Work out the finished part from the listing and answer in its coordinate system (mm). Give positions to 0.01 mm unless a question says otherwise; leave off trailing zeros. Order: outer loops, then holes, each group sorted by start corner. A loop starts at its lowest first (then second) coordinate and runs counter-clockwise, first axis right, second up. Notation, with made-up numbers: (10, 11.5) -> (49, 11.5) arc R9 ccw to (49, 15.5) -> close; hole circle Ø1 at (18.5, -20). An arc over 180 degrees is marked (long way). Answer as CSV lines item,"result". Start each with the question number.
1. For a pull along Y with two mould halves and no side action, classify faces 1 (the flat face through (110, -9, 1.016)), 2 (the flat face through (12, 29, 0.508)) as released by +Y, released by -Y, zero draft, split by the parting line, or undercut.
2. Find the intervals of material crossed by L1, parallel to Y at x = 28.5, z = 0.55; L2, parallel to Z at x = 58, y = 4, in increasing order.
3. A flat-ended cylindrical pin translates along its axis: pin 1 (0.6 mm diameter, centred on x = -53.5, z = 1, fed in from -Y). Find the tip coordinate at first contact, or state that the pin passes through.
4. A cutting plane is placed at B-B (z = 0.7). State how many separate pieces and enclosed holes the cut face has, then the cut area to 3 significant figures.
5. A cutting plane is placed at A-A (x = -7.5). Give the vertices of the cut face in (y, z), then the cut area to 3 significant figures.
from build123d import *

# Parameters (mm, degrees)
F0_W     = 226.06
F0_H     = 142.24
F0_W_2   = 25.4
F0_H_2   = 25.4
F1_DEPTH = 0.508
F2_DEPTH = 1.016


with BuildPart() as f1:
    # F0 (on Top) → F1 (new body)
    with BuildSketch(Plane.XY):
        with Locations((12.174503, 18.332164)):
            Rectangle(F0_W, F0_H)
        with Locations((-85.615497, -37.547836)):
            Rectangle(F0_W_2, F0_H_2, mode=Mode.SUBTRACT)
        with Locations((-57.675497, -37.547836)):
            Rectangle(F0_W_2, F0_H_2, mode=Mode.SUBTRACT)
        with Locations((-29.735497, -37.547836)):
            Rectangle(F0_W_2, F0_H_2, mode=Mode.SUBTRACT)
        with Locations((-1.795497, -37.547836)):
            Rectangle(F0_W_2, F0_H_2, mode=Mode.SUBTRACT)
        with Locations((-85.615497, -9.607836)):
            Rectangle(F0_W_2, F0_H_2, mode=Mode.SUBTRACT)
        with Locations((-57.675497, -9.607836)):
            Rectangle(F0_W_2, F0_H_2, mode=Mode.SUBTRACT)
        with Locations((-85.615497, 18.332164)):
            Rectangle(F0_W_2, F0_H_2, mode=Mode.SUBTRACT)
        with Locations((-57.675497, 18.332164)):
            Rectangle(F0_W_2, F0_H_2, mode=Mode.SUBTRACT)
        with Locations((-29.735497, -9.607836)):
            Rectangle(F0_W_2, F0_H_2, mode=Mode.SUBTRACT)
        with Locations((-1.795497, -9.607836)):
            Rectangle(F0_W_2, F0_H_2, mode=Mode.SUBTRACT)
        with Locations((-29.735497, 18.332164)):
            Rectangle(F0_W_2, F0_H_2, mode=Mode.SUBTRACT)
        with Locations((-1.795497, 18.332164)):
            Rectangle(F0_W_2, F0_H_2, mode=Mode.SUBTRACT)
        with Locations((26.144503, -37.547836)):
            Rectangle(F0_W_2, F0_H_2, mode=Mode.SUBTRACT)
        with Locations((54.084503, -37.547836)):
            Rectangle(F0_W_2, F0_H_2, mode=Mode.SUBTRACT)
        with Locations((82.024503, -37.547836)):
            Rectangle(F0_W_2, F0_H_2, mode=Mode.SUBTRACT)
        with Locations((109.964503, -37.547836)):
            Rectangle(F0_W_2, F0_H_2, mode=Mode.SUBTRACT)
        with Locations((26.144503, -9.607836)):
            Rectangle(F0_W_2, F0_H_2, mode=Mode.SUBTRACT)
        with Locations((54.084503, -9.607836)):
            Rectangle(F0_W_2, F0_H_2, mode=Mode.SUBTRACT)
        with Locations((26.144503, 18.332164)):
            Rectangle(F0_W_2, F0_H_2, mode=Mode.SUBTRACT)
        with Locations((54.084503, 18.332164)):
            Rectangle(F0_W_2, F0_H_2, mode=Mode.SUBTRACT)
        with Locations((82.024503, -9.607836)):
            Rectangle(F0_W_2, F0_H_2, mode=Mode.SUBTRACT)
        with Locations((109.964503, -9.607836)):
            Rectangle(F0_W_2, F0_H_2, mode=Mode.SUBTRACT)
        with Locations((82.024503, 18.332164)):
            Rectangle(F0_W_2, F0_H_2, mode=Mode.SUBTRACT)
        with Locations((109.964503, 18.332164)):
            Rectangle(F0_W_2, F0_H_2, mode=Mode.SUBTRACT)
        with Locations((-85.615497, 46.272164)):
            Rectangle(F0_W_2, F0_H_2, mode=Mode.SUBTRACT)
        with Locations((-57.675497, 46.272164)):
            Rectangle(F0_W_2, F0_H_2, mode=Mode.SUBTRACT)
        with Locations((-29.735497, 46.272164)):
            Rectangle(F0_W_2, F0_H_2, mode=Mode.SUBTRACT)
        with Locations((-1.795497, 46.272164)):
            Rectangle(F0_W_2, F0_H_2, mode=Mode.SUBTRACT)
        with Locations((-85.615497, 74.212164)):
            Rectangle(F0_W_2, F0_H_2, mode=Mode.SUBTRACT)
        with Locations((-57.675497, 74.212164)):
            Rectangle(F0_W_2, F0_H_2, mode=Mode.SUBTRACT)
        with Locations((-29.735497, 74.212164)):
            Rectangle(F0_W_2, F0_H_2, mode=Mode.SUBTRACT)
        with Locations((-1.795497, 74.212164)):
            Rectangle(F0_W_2, F0_H_2, mode=Mode.SUBTRACT)
        with Locations((26.144503, 46.272164)):
            Rectangle(F0_W_2, F0_H_2, mode=Mode.SUBTRACT)
        with Locations((54.084503, 46.272164)):
            Rectangle(F0_W_2, F0_H_2, mode=Mode.SUBTRACT)
        with Locations((82.024503, 46.272164)):
            Rectangle(F0_W_2, F0_H_2, mode=Mode.SUBTRACT)
        with Locations((109.964503, 46.272164)):
            Rectangle(F0_W_2, F0_H_2, mode=Mode.SUBTRACT)
        with Locations((26.144503, 74.212164)):
            Rectangle(F0_W_2, F0_H_2, mode=Mode.SUBTRACT)
        with Locations((54.084503, 74.212164)):
            Rectangle(F0_W_2, F0_H_2, mode=Mode.SUBTRACT)
        with Locations((82.024503, 74.212164)):
            Rectangle(F0_W_2, F0_H_2, mode=Mode.SUBTRACT)
        with Locations((109.964503, 74.212164)):
            Rectangle(F0_W_2, F0_H_2, mode=Mode.SUBTRACT)
    extrude(amount=F1_DEPTH)

    # F0 (on Top) → F2 (join)
    with BuildSketch(Plane.XY):
        with Locations((-85.615497, 18.332164)):
            Rectangle(F0_W_2, F0_H_2)
        with Locations((-57.675497, 18.332164)):
            Rectangle(F0_W_2, F0_H_2)
        with Locations((-57.675497, 46.272164)):
            Rectangle(F0_W_2, F0_H_2)
        with Locations((-85.615497, 46.272164)):
            Rectangle(F0_W_2, F0_H_2)
        with Locations((-85.615497, 74.212164)):
            Rectangle(F0_W_2, F0_H_2)
        with Locations((-57.675497, 74.212164)):
            Rectangle(F0_W_2, F0_H_2)
        with Locations((-85.615497, -9.607836)):
            Rectangle(F0_W_2, F0_H_2)
        with Locations((-57.675497, -9.607836)):
            Rectangle(F0_W_2, F0_H_2)
        with Locations((-57.675497, -37.547836)):
            Rectangle(F0_W_2, F0_H_2)
        with Locations((-85.615497, -37.547836)):
            Rectangle(F0_W_2, F0_H_2)
        with Locations((-29.735497, -37.547836)):
            Rectangle(F0_W_2, F0_H_2)
        with Locations((-29.735497, -9.607836)):
            Rectangle(F0_W_2, F0_H_2)
        with Locations((-29.735497, 18.332164)):
            Rectangle(F0_W_2, F0_H_2)
        with Locations((-29.735497, 46.272164)):
            Rectangle(F0_W_2, F0_H_2)
        with Locations((-29.735497, 74.212164)):
            Rectangle(F0_W_2, F0_H_2)
        with Locations((-1.795497, 74.212164)):
            Rectangle(F0_W_2, F0_H_2)
        with Locations((-1.795497, 46.272164)):
            Rectangle(F0_W_2, F0_H_2)
        with Locations((-1.795497, 18.332164)):
            Rectangle(F0_W_2, F0_H_2)
        with Locations((-1.795497, -9.607836)):
            Rectangle(F0_W_2, F0_H_2)
        with Locations((-1.795497, -37.547836)):
            Rectangle(F0_W_2, F0_H_2)
        with Locations((26.144503, -37.547836)):
            Rectangle(F0_W_2, F0_H_2)
        with Locations((26.144503, -9.607836)):
            Rectangle(F0_W_2, F0_H_2)
        with Locations((26.144503, 18.332164)):
            Rectangle(F0_W_2, F0_H_2)
        with Locations((26.144503, 46.272164)):
            Rectangle(F0_W_2, F0_H_2)
        with Locations((26.144503, 74.212164)):
            Rectangle(F0_W_2, F0_H_2)
        with Locations((54.084503, 74.212164)):
            Rectangle(F0_W_2, F0_H_2)
        with Locations((54.084503, 46.272164)):
            Rectangle(F0_W_2, F0_H_2)
        with Locations((54.084503, 18.332164)):
            Rectangle(F0_W_2, F0_H_2)
        with Locations((54.084503, -9.607836)):
            Rectangle(F0_W_2, F0_H_2)
        with Locations((54.084503, -37.547836)):
            Rectangle(F0_W_2, F0_H_2)
        with Locations((82.024503, -37.547836)):
            Rectangle(F0_W_2, F0_H_2)
        with Locations((82.024503, -9.607836)):
            Rectangle(F0_W_2, F0_H_2)
        with Locations((82.024503, 18.332164)):
            Rectangle(F0_W_2, F0_H_2)
        with Locations((82.024503, 46.272164)):
            Rectangle(F0_W_2, F0_H_2)
        with Locations((82.024503, 74.212164)):
            Rectangle(F0_W_2, F0_H_2)
        with Locations((109.964503, 74.212164)):
            Rectangle(F0_W_2, F0_H_2)
        with Locations((109.964503, 46.272164)):
            Rectangle(F0_W_2, F0_H_2)
        with Locations((109.964503, 18.332164)):
            Rectangle(F0_W_2, F0_H_2)
        with Locations((109.964503, -9.607836)):
            Rectangle(F0_W_2, F0_H_2)
        with Locations((109.964503, -37.547836)):
            Rectangle(F0_W_2, F0_H_2)
    extrude(amount=F2_DEPTH)


solid = f1.part
Answer sheet:
1,face 1,"zero draft"
1,face 2,"undercut"
2,L1,"y = -50.25 to -24.85, -22.31 to 3.09, 5.63 to 31.03, 33.57 to 58.97, 61.51 to 86.91"
2,L2,"z = 0 to 0.51"
3,pin 1,"stops at y = -50.25"
4,separate pieces,"40"
4,enclosed holes,"0"
4,area,"25,800 mm^2"
5,outline,"(-52.79, 0) -> (89.45, 0) -> (89.45, 0.51) -> (86.91, 0.51) -> (86.91, 1.02) -> (61.51, 1.02) -> (61.51, 0.51) -> (58.97, 0.51) -> (58.97, 1.02) -> (33.57, 1.02) -> (33.57, 0.51) -> (31.03, 0.51) -> (31.03, 1.02) -> (5.63, 1.02) -> (5.63, 0.51) -> (3.09, 0.51) -> (3.09, 1.02) -> (-22.31, 1.02) -> (-22.31, 0.51) -> (-24.85, 0.51) -> (-24.85, 1.02) -> (-50.25, 1.02) -> (-50.25, 0.51) -> (-52.79, 0.51) -> close"
5,area,"137 mm^2"
